from build123d import *

# Parameters (mm, degrees)
F2_T = 2.5


# Not quite as in the source:
# - a shell that OpenCascade refuses in one call is made with other operations: the cavity is built on its own and cut out


with BuildPart() as f1:
    # F0 (on Front) → F1 (revolve)
    with BuildSketch(Plane.XZ):
        with BuildLine():
            Line((-96.4535274908, 0), (81.0464725092, 0))
            Line((81.0464725092, 0), (81.0464725092, 27.5))
            Line((81.0464725092, 27.5), (78.0464725092, 27.5))
            Line((78.0464725092, 27.5), (78.0464725092, 27))
            Line((78.0464725092, 27), (76.0464725092, 27))
            Line((76.0464725092, 27), (76.0464725092, 27.5))
            Line((76.0464725092, 27.5), (72.0464725092, 27.5))
            Line((72.0464725092, 27.5), (72.0464725092, 27))
            Line((72.0464725092, 27), (70.0464725092, 27))
            Line((70.0464725092, 27), (70.0464725092, 27.5))
            Line((70.0464725092, 27.5), (66.0464725092, 27.5))
            Line((66.0464725092, 27.5), (66.0464725092, 27))
            Line((66.0464725092, 27), (64.0464725092, 27))
            Line((64.0464725092, 27), (64.0464725092, 27.5))
            Line((64.0464725092, 27.5), (60.0464725092, 27.5))
            Line((60.0464725092, 27.5), (60.0464725092, 27))
            Line((60.0464725092, 27), (58.0464725092, 27))
            Line((58.0464725092, 27), (58.0464725092, 27.5))
            Line((58.0464725092, 27.5), (56.0464725092, 27.5))
            Line((56.0464725092, 27.5), (54.0464725092, 27.5))
            Line((54.0464725092, 27.5), (54.0464725092, 27))
            Line((54.0464725092, 27), (52.0464725092, 27))
            Line((52.0464725092, 27), (52.0464725092, 27.5))
            Line((52.0464725092, 27.5), (48.0464725092, 27.5))
            Line((48.0464725092, 27.5), (48.0464725092, 27))
            Line((48.0464725092, 27), (46.0464725092, 27))
            Line((46.0464725092, 27), (46.0464725092, 27.5))
            Line((46.0464725092, 27.5), (42.0464725092, 27.5))
            Line((42.0464725092, 27.5), (42.0464725092, 27))
            Line((42.0464725092, 27), (40.0464725092, 27))
            Line((40.0464725092, 27), (40.0464725092, 27.5))
            Line((40.0464725092, 27.5), (36.0464725092, 27.5))
            Line((36.0464725092, 27.5), (36.0464725092, 27))
            Line((36.0464725092, 27), (34.0464725092, 27))
            Line((34.0464725092, 27), (34.0464725092, 27.5))
            Line((34.0464725092, 27.5), (32.0464725092, 27.5))
            Line((32.0464725092, 27.5), (25.0464725092, 27.5))
            Line((25.0464725092, 27.5), (-68.9535274908, 27.5))
            ThreePointArc((-68.9535274908, 27.5), (-88.3989639735, 19.4454364826), (-96.4535274908, 0))
        make_face()
    revolve(axis=Axis((-7.7035274908, 0, 0), (-1, 0, 0)))

    # F2: shell of thickness 2.5, made by hand


with BuildPart() as f2_core1:
    # F2_t2: copy of F1
    add(f1.part)

    # the walls: a layer under each face that stays
    f2_faces = [f2_core1.faces().sort_by_distance(p)[0] for p in [
        (-88.3989639735, 0, -19.4454364826),
        (-17.4535274908, 0, -27.5),
        (34.0464725092, -13.2407407407, -24.0625),
        (35.0464725092, 0, -27),
        (36.0464725092, -13.2407407407, 24.0625),
        (38.0464725092, 0, -27.5),
        (40.0464725092, -13.2407407407, -24.0625),
        (41.0464725092, 0, -27),
        (42.0464725092, -13.2407407407, 24.0625),
        (44.0464725092, 0, -27.5),
        (46.0464725092, -13.2407407407, -24.0625),
        (47.0464725092, 0, -27),
        (48.0464725092, -13.2407407407, 24.0625),
        (50.0464725092, 0, -27.5),
        (52.0464725092, -13.2407407407, -24.0625),
        (53.0464725092, 0, -27),
        (54.0464725092, -13.2407407407, 24.0625),
        (56.0464725092, 0, -27.5),
        (58.0464725092, -13.2407407407, -24.0625),
        (59.0464725092, 0, -27),
        (60.0464725092, -13.2407407407, 24.0625),
        (62.0464725092, 0, -27.5),
        (64.0464725092, -13.2407407407, -24.0625),
        (65.0464725092, 0, -27),
        (66.0464725092, -13.2407407407, 24.0625),
        (68.0464725092, 0, -27.5),
        (70.0464725092, -13.2407407407, -24.0625),
        (71.0464725092, 0, -27),
        (72.0464725092, -13.2407407407, 24.0625),
        (74.0464725092, 0, -27.5),
        (76.0464725092, -13.2407407407, -24.0625),
        (77.0464725092, 0, -27),
        (78.0464725092, -13.2407407407, 24.0625),
        (79.5464725092, 0, -27.5),
    ]]
    thicken(f2_faces, amount=-F2_T, mode=Mode.SUBTRACT)

    # F2_s3 → F2_t4 (revolve, cut)
    with BuildSketch(Plane.XZ):
        Polygon((34.0714725092, 27.025), (31.5464725092, 27), (31.5464725092, 24.5), (34.0464725092, 24.5), align=None)
    revolve(axis=Axis((34.0464725092, 0, 0), (-1, 0, 0)), mode=Mode.SUBTRACT)

    # F2_s5 → F2_t6 (revolve, cut)
    with BuildSketch(Plane.XZ):
        Polygon((36.0214725092, 27.025), (36.0464725092, 24.5), (38.5464725092, 24.5), (38.5464725092, 27), align=None)
    revolve(axis=Axis((36.0464725092, 0, 0), (-1, 0, 0)), mode=Mode.SUBTRACT)

    # F2_s7 → F2_t8 (revolve, cut)
    with BuildSketch(Plane.XZ):
        Polygon((40.0714725092, 27.025), (37.5464725092, 27), (37.5464725092, 24.5), (40.0464725092, 24.5), align=None)
    revolve(axis=Axis((40.0464725092, 0, 0), (-1, 0, 0)), mode=Mode.SUBTRACT)

    # F2_s9 → F2_t10 (revolve, cut)
    with BuildSketch(Plane.XZ):
        Polygon((42.0214725092, 27.025), (42.0464725092, 24.5), (44.5464725092, 24.5), (44.5464725092, 27), align=None)
    revolve(axis=Axis((42.0464725092, 0, 0), (-1, 0, 0)), mode=Mode.SUBTRACT)

    # F2_s11 → F2_t12 (revolve, cut)
    with BuildSketch(Plane.XZ):
        Polygon((46.0714725092, 27.025), (43.5464725092, 27), (43.5464725092, 24.5), (46.0464725092, 24.5), align=None)
    revolve(axis=Axis((46.0464725092, 0, 0), (-1, 0, 0)), mode=Mode.SUBTRACT)

    # F2_s13 → F2_t14 (revolve, cut)
    with BuildSketch(Plane.XZ):
        Polygon((48.0214725092, 27.025), (48.0464725092, 24.5), (50.5464725092, 24.5), (50.5464725092, 27), align=None)
    revolve(axis=Axis((48.0464725092, 0, 0), (-1, 0, 0)), mode=Mode.SUBTRACT)

    # F2_s15 → F2_t16 (revolve, cut)
    with BuildSketch(Plane.XZ):
        Polygon((52.0714725092, 27.025), (49.5464725092, 27), (49.5464725092, 24.5), (52.0464725092, 24.5), align=None)
    revolve(axis=Axis((52.0464725092, 0, 0), (-1, 0, 0)), mode=Mode.SUBTRACT)

    # F2_s17 → F2_t18 (revolve, cut)
    with BuildSketch(Plane.XZ):
        Polygon((54.0214725092, 27.025), (54.0464725092, 24.5), (56.5464725092, 24.5), (56.5464725092, 27), align=None)
    revolve(axis=Axis((54.0464725092, 0, 0), (-1, 0, 0)), mode=Mode.SUBTRACT)

    # F2_s19 → F2_t20 (revolve, cut)
    with BuildSketch(Plane.XZ):
        Polygon((58.0714725092, 27.025), (55.5464725092, 27), (55.5464725092, 24.5), (58.0464725092, 24.5), align=None)
    revolve(axis=Axis((58.0464725092, 0, 0), (-1, 0, 0)), mode=Mode.SUBTRACT)

    # F2_s21 → F2_t22 (revolve, cut)
    with BuildSketch(Plane.XZ):
        Polygon((60.0214725092, 27.025), (60.0464725092, 24.5), (62.5464725092, 24.5), (62.5464725092, 27), align=None)
    revolve(axis=Axis((60.0464725092, 0, 0), (-1, 0, 0)), mode=Mode.SUBTRACT)

    # F2_s23 → F2_t24 (revolve, cut)
    with BuildSketch(Plane.XZ):
        Polygon((64.0714725092, 27.025), (61.5464725092, 27), (61.5464725092, 24.5), (64.0464725092, 24.5), align=None)
    revolve(axis=Axis((64.0464725092, 0, 0), (-1, 0, 0)), mode=Mode.SUBTRACT)

    # F2_s25 → F2_t26 (revolve, cut)
    with BuildSketch(Plane.XZ):
        Polygon((66.0214725092, 27.025), (66.0464725092, 24.5), (68.5464725092, 24.5), (68.5464725092, 27), align=None)
    revolve(axis=Axis((66.0464725092, 0, 0), (-1, 0, 0)), mode=Mode.SUBTRACT)

    # F2_s27 → F2_t28 (revolve, cut)
    with BuildSketch(Plane.XZ):
        Polygon((70.0714725092, 27.025), (67.5464725092, 27), (67.5464725092, 24.5), (70.0464725092, 24.5), align=None)
    revolve(axis=Axis((70.0464725092, 0, 0), (-1, 0, 0)), mode=Mode.SUBTRACT)

    # F2_s29 → F2_t30 (revolve, cut)
    with BuildSketch(Plane.XZ):
        Polygon((72.0214725092, 27.025), (72.0464725092, 24.5), (74.5464725092, 24.5), (74.5464725092, 27), align=None)
    revolve(axis=Axis((72.0464725092, 0, 0), (-1, 0, 0)), mode=Mode.SUBTRACT)

    # F2_s31 → F2_t32 (revolve, cut)
    with BuildSketch(Plane.XZ):
        Polygon((76.0714725092, 27.025), (73.5464725092, 27), (73.5464725092, 24.5), (76.0464725092, 24.5), align=None)
    revolve(axis=Axis((76.0464725092, 0, 0), (-1, 0, 0)), mode=Mode.SUBTRACT)

    # F2_s33 → F2_t34 (revolve, cut)
    with BuildSketch(Plane.XZ):
        Polygon((78.0214725092, 27.025), (78.0464725092, 24.5), (80.5464725092, 24.5), (80.5464725092, 27), align=None)
    revolve(axis=Axis((78.0464725092, 0, 0), (-1, 0, 0)), mode=Mode.SUBTRACT)


with BuildPart() as f1_1:
    add(f1.part)

    # what is left inside the walls is the cavity
    f2_cavity = [f2_core1.part.solids().sort_by_distance(p)[0] for p in [
        (-1.953527, 0, -24.975),
    ]]
    add(f2_cavity, mode=Mode.SUBTRACT)


solid = f1_1.part
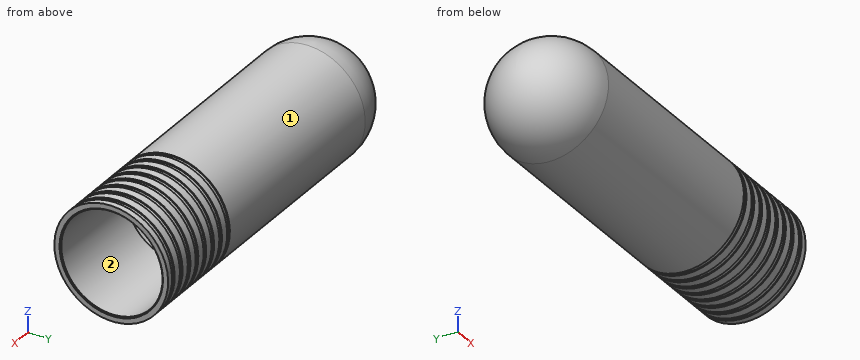
Here's how the part is built. I have some questions about the finished solid (model axes, mm). Face numbers are marked on the shaded views. Coordinates: 2 decimals unless noted, no trailing zeros. Loops run counter-clockwise (first coordinate to the right, second up) from the corner with the lowest first, then second, coordinate; pieces in that order, holes last. Notation, with made-up numbers: (63.25, -22) -> (79.25, -22) arc R19 cw to (79.25, -3) -> close; hole circle Ø11 at (-12, 62.5). An arc over 180 degrees is marked (long way). Use one line per item in the form item = value. Start each with the question number.
(1) Will these pins go through, and if not, where does the flat tip stop? pin 1 (16.5 mm diameter, centred on y = 9, z = 8, fed in from +X); pin 2 (25 mm diameter, centred on y = -2.5, z = 12.5, fed in from +X); pin 3 (3 mm diameter, centred on x = 59, z = -9, fed in from +Y); pin 4 (3 mm diameter, centred on x = -37.5, z = -5.5, fed in from +Y).
(2) If we section it at A-A (x = -29): Please give me the cut outline in (y, z).
(3) We'd pull the mould along Z, two halves only. Please class the marked faces 1 and 2: pulls with the +Z half, pulls with the -Z half, needs draft (parallel to the pull), parting line crosses it, or undercut.
(4) Please list where these lines run through material, in increasing order: line 1 along Y through (x, z) = (6, 0); line 2 along Z through (x, y) = (-87, -13.5); line 3 along Z through (x, y) = (-78, 18.5).
Verdict:
q1.pin_1 = -83.56
q1.pin_2 = 81.05
q1.pin_3 = 26.36
q1.pin_4 = 27.21
q2.outline = circle Ø55 at (0, 0); hole circle Ø50 at (0, 0)
q3.face_1 = parting line crosses it
q3.face_2 = undercut
q4.line_1 = -27.5 to -25, 25 to 27.5
q4.line_2 = -15.76 to -10.82, 10.82 to 15.76
q4.line_3 = -18.23 to -14.17, 14.17 to 18.23
